```python
from build123d import *

# Parameters (mm, degrees)
F0_R      = 30.39041
F1_DEPTH  = 43.688
F3_DEPTH  = 17.78
F5_DEPTH  = 17.78
F6_R      = 8.542504
F7_DEPTH  = 104.14
F8_R      = 26.119062
F9_DEPTH  = 17.78
F10_R     = 26.864742
F11_DEPTH = 17.78
F12_R     = 7.954549
F13_DEPTH = 97.79


with BuildPart() as f1:
    # F0 (on Front) → F1 (new body, symmetric)
    with BuildSketch(Plane.XZ):
        Circle(F0_R)
    extrude(amount=F1_DEPTH, both=True)

    # F2 (on face) → F3 (join)
    with BuildSketch(Plane.XZ.offset(43.688)):
        with BuildLine():
            Line((-25.588728, 54.975592), (-25.588728, 16.394938))
            ThreePointArc((-25.588728, 16.394938), (0, 30.39041), (25.588728, 16.394938))
            Line((25.588728, 16.394938), (25.588728, 54.975592))
            Line((25.588728, 54.975592), (-25.588728, 54.975592))
        make_face()
        with BuildLine():
            Line((-25.588728, 16.394938), (-25.588728, -16.394938))
            Line((-25.588728, -16.394938), (25.588728, -16.394938))
            Line((25.588728, -16.394938), (25.588728, 16.394938))
            ThreePointArc((25.588728, 16.394938), (0, 30.39041), (-25.588728, 16.394938))
        make_face()
    extrude(amount=-F3_DEPTH)

    # F4 (on face) → F5 (join)
    with BuildSketch(Plane(origin=(0, 43.688, 0), x_dir=(-1, 0, 0), z_dir=(0, 1, 0))):
        with BuildLine():
            Line((-26.646163, 55.732163), (-26.646163, 14.613658))
            ThreePointArc((-26.646163, 14.613658), (0, 30.39041), (26.646163, 14.613658))
            Line((26.646163, 14.613658), (26.646163, 55.732163))
            Line((26.646163, 55.732163), (-26.646163, 55.732163))
        make_face()
        with BuildLine():
            Line((-26.646163, 14.613658), (-26.646163, -14.613658))
            Line((-26.646163, -14.613658), (26.646163, -14.613658))
            Line((26.646163, -14.613658), (26.646163, 14.613658))
            ThreePointArc((26.646163, 14.613658), (0, 30.39041), (-26.646163, 14.613658))
        make_face()
    extrude(amount=-F5_DEPTH)

    # F6 (on face) → F7 (cut)
    with BuildSketch(Plane(origin=(0, 43.688, 0), x_dir=(-1, 0, 0), z_dir=(0, 1, 0))):
        Circle(F6_R)
    extrude(amount=-F7_DEPTH, mode=Mode.SUBTRACT)

    # F8 (on face) → F9 (join)
    with BuildSketch(Plane.XZ.offset(43.688)):
        with Locations((0, 50.235286)):
            Circle(F8_R)
    extrude(amount=-F9_DEPTH)

    # F10 (on face) → F11 (join)
    with BuildSketch(Plane(origin=(0, 43.688, 0), x_dir=(-1, 0, 0), z_dir=(0, 1, 0))):
        with Locations((0, 49.751956)):
            Circle(F10_R)
    extrude(amount=-F11_DEPTH)

    # F12 (on face) → F13 (cut)
    with BuildSketch(Plane(origin=(0, 43.688, 0), x_dir=(-1, 0, 0), z_dir=(0, 1, 0))):
        with Locations((0, 49.751956)):
            Circle(F12_R)
    extrude(amount=-F13_DEPTH, mode=Mode.SUBTRACT)


solid = f1.part
```
Design review of the part built by this model. Coordinates are the model's own, in mm. A direction names the side the tool comes from. Give positions to 0.01 mm unless a question says otherwise; leave off trailing zeros. Order: outer loops, then holes, each group sorted by start corner. A loop starts at its lowest first (then second) coordinate and runs counter-clockwise, first axis right, second up. Notation, with made-up numbers: (11.5, 18.25) - (52.5, 18.25) arc R29 ccw to (52.5, 53.25) - close; hole circle Ø7 at (24, 76.25). An arc over 180 degrees is marked (long way). Use a Markdown table: item, result. Add a question column.
(1) Machinability: for faces 1 (the face through (26.646, 35, 31)), 2 (the face through (-25.589, -35, 31)), 3 (the face through (-26.646, 35, 30)), 4 (the face through (-26.646, 35, 54)), 5 (the face through (26.646, 35, 54)), which of the approach directions +Z, -Z, +X, -X, +Y, -Y give a long, thin tool a straight path to every point of the face, cutting with its end or side? Answer none if there is none.
(2) Add section C-C on y = 10. Give the boundary of the cut face in (x, z) (1 decimal), then the cut area to 3 significant figures.
(3) Clearance check with flat-ended pins moving along their axes: P1, Ø5.5, axis at y = 35.5, z = 25.5, coming from the +X side; P2, Ø18.5, axis at x = 0, z = 49.75, coming from the +Y side; P3, Ø6, axis at y = -25, z = 54.5, coming from the -X side; P4, Ø0.8, axis at y = 39, z = 55, coming from the -X side. State where each tip first meets the part, or that it passes through.
(4) Add section D-D on z = 34. Give the boundary of the cut face in (x, y), then the cut area to 3 significant figures.
(5) Add section A-A on x = 0. Give the boundary of the cut face in (y, z).
(6) Mouldability with a two-part tool opening along Z and no side actions: class faces 6 (the face through (1.724, 34.922, 41.987)), 7 (the face through (-0.51, 34.92, 76.61)), 8 (the face through (0, -25.908, 40)) as +Z half, -Z half, draft (parallel to the pull), parting line (faces both ways), or undercut.
(7) Wall thickness on probe 1 along Z at (x, y) = (0, -32.75); probe 2 along Z at (x, y) = (0, 33.75); probe 3 along Y at (x, z) = (-12, 32.5): over which ranges is each line inside the solid? List them lowest first. Write a range as [from, to].
(8) Add section B-B on z = 0. Give the boundary of the cut face in (x, y), then the cut area to 3 significant figures.
Report:
| question | item | result |
|---|---|---|
| 1 | face 1 | +X, +Y, -Y |
| 1 | face 2 | -X, -Y |
| 1 | face 3 | -X, +Y, -Y |
| 1 | face 4 | +Z, -X, +Y, -Y |
| 1 | face 5 | +Z, +X, +Y, -Y |
| 2 | outline | circle Ø60.8 at (0, 0); hole circle Ø17.1 at (0, 0) |
| 2 | area | 2,670 mm² |
| 3 | P1 | stops at x = 26.65 |
| 3 | P2 | stops at y = 43.69 |
| 3 | P3 | stops at x = -26.08 |
| 3 | P4 | stops at x = -26.65 |
| 4 | outline | (-26.65, 25.91) - (26.65, 25.91) - (26.65, 43.69) - (-26.65, 43.69) - close; (-25.59, -43.69) - (25.59, -43.69) - (25.59, -25.91) - (-25.59, -25.91) - close |
| 4 | area | 1,860 mm² |
| 5 | outline | (-43.69, -30.39) - (43.69, -30.39) - (43.69, -8.54) - (-43.69, -8.54) - close; (-43.69, 8.54) - (43.69, 8.54) - (43.69, 41.8) - (25.91, 41.8) - (25.91, 30.39) - (-25.91, 30.39) - (-25.91, 41.8) - (-43.69, 41.8) - close; (-43.69, 57.71) - (-25.91, 57.71) - (-25.91, 76.35) - (-43.69, 76.35) - close; (25.91, 57.71) - (43.69, 57.71) - (43.69, 76.62) - (25.91, 76.62) - close |
| 6 | face 6 | undercut |
| 6 | face 7 | +Z half |
| 6 | face 8 | draft |
| 7 | probe 1 | z = [-30.39, -8.54], [8.54, 41.8], [57.71, 76.35] |
| 7 | probe 2 | z = [-30.39, -8.54], [8.54, 41.8], [57.71, 76.62] |
| 7 | probe 3 | y = [-43.69, -25.91], [25.91, 43.69] |
| 8 | outline | (-30.39, -43.69) - (-8.54, -43.69) - (-8.54, 43.69) - (-30.39, 43.69) - close; (8.54, -43.69) - (30.39, -43.69) - (30.39, 43.69) - (8.54, 43.69) - close |
| 8 | area | 3,820 mm² |
